from build123d import *

# Parameters (mm, degrees)
EXTRUDE7_START     = 10
SKETCH1_R          = 2.25
SKETCH1_R_2        = 14.05
EXTRUDE7_DEPTH     = 30
CUT_EXTRUDE6_START = 2
SKETCH8_R          = 2.25
CUT_EXTRUDE6_DEPTH = 30


with BuildPart() as part:
    # Sketch1 → Extrude7 (new body)
    with BuildSketch(Plane.XY.offset(EXTRUDE7_START)):
        Polygon((20, 44), (-20, 44), (-22, 44), (-22, -44), (-20, -44), (20, -44), align=None)
        with Locations((-13.435028843, -13.435028843)):
            Circle(SKETCH1_R, mode=Mode.SUBTRACT)
        with Locations((0, -19)):
            Circle(SKETCH1_R, mode=Mode.SUBTRACT)
        with Locations((13.435028843, -13.435028843)):
            Circle(SKETCH1_R, mode=Mode.SUBTRACT)
        with Locations((-13.435028843, 13.435028843)):
            Circle(SKETCH1_R, mode=Mode.SUBTRACT)
        Circle(SKETCH1_R_2, mode=Mode.SUBTRACT)
        with Locations((0, 19)):
            Circle(SKETCH1_R, mode=Mode.SUBTRACT)
        with Locations((13.435028843, 13.435028843)):
            Circle(SKETCH1_R, mode=Mode.SUBTRACT)
        Polygon((20, 44), (-20, 44), (-22, 44), (-22, -44), (-20, -44), (20, -44), align=None)
        with Locations((-13.435028843, -13.435028843)):
            Circle(SKETCH1_R, mode=Mode.SUBTRACT)
        with Locations((0, -19)):
            Circle(SKETCH1_R, mode=Mode.SUBTRACT)
        with Locations((13.435028843, -13.435028843)):
            Circle(SKETCH1_R, mode=Mode.SUBTRACT)
        with Locations((-13.435028843, 13.435028843)):
            Circle(SKETCH1_R, mode=Mode.SUBTRACT)
        Circle(SKETCH1_R_2, mode=Mode.SUBTRACT)
        with Locations((0, 19)):
            Circle(SKETCH1_R, mode=Mode.SUBTRACT)
        with Locations((13.435028843, 13.435028843)):
            Circle(SKETCH1_R, mode=Mode.SUBTRACT)
        Polygon((20, 44), (-20, 44), (-22, 44), (-22, -44), (-20, -44), (20, -44), align=None)
        with Locations((-13.435028843, -13.435028843)):
            Circle(SKETCH1_R, mode=Mode.SUBTRACT)
        with Locations((0, -19)):
            Circle(SKETCH1_R, mode=Mode.SUBTRACT)
        with Locations((13.435028843, -13.435028843)):
            Circle(SKETCH1_R, mode=Mode.SUBTRACT)
        with Locations((-13.435028843, 13.435028843)):
            Circle(SKETCH1_R, mode=Mode.SUBTRACT)
        Circle(SKETCH1_R_2, mode=Mode.SUBTRACT)
        with Locations((0, 19)):
            Circle(SKETCH1_R, mode=Mode.SUBTRACT)
        with Locations((13.435028843, 13.435028843)):
            Circle(SKETCH1_R, mode=Mode.SUBTRACT)
    extrude(amount=EXTRUDE7_DEPTH)

    # Sketch8 → Cut-Extrude6 (cut)
    with BuildSketch(Plane.ZY.offset(20).offset(CUT_EXTRUDE6_START)):
        with Locations((17.5, 39)):
            Circle(SKETCH8_R)
        with Locations((32.5, 39)):
            Circle(SKETCH8_R)
        with Locations((17.5, -39)):
            Circle(SKETCH8_R)
        with Locations((32.5, -39)):
            Circle(SKETCH8_R)
        with Locations((17.5, 29)):
            Circle(SKETCH8_R)
        with Locations((32.5, 29)):
            Circle(SKETCH8_R)
        with Locations((17.5, -29)):
            Circle(SKETCH8_R)
        with Locations((32.5, -29)):
            Circle(SKETCH8_R)
    extrude(amount=-CUT_EXTRUDE6_DEPTH, mode=Mode.SUBTRACT)


solid = part.part
Work out the finished part from the listing and answer in its coordinate system (mm). A direction names the side the tool comes from. Coordinates: 2 decimals unless noted, no trailing zeros. Write each loop counter-clockwise with the first axis right and the second up, starting at its lowest first coordinate (ties: lowest second). Pieces come first, ordered by that corner, then holes. Notation, with made-up numbers: M -7,-4.5 L 8,-4.5 A25 cw 8,34.5 Z; hole C 79,1.5 d6. An arc over 180 degrees is marked long. Write item = value, one per line.
1. Flat-ended cylindrical pins translate along their axes: pin 1 (4 mm diameter, centred on x = 13.44, y = -13.44, fed in from -Z); pin 2 (2.5 mm diameter, centred on y = 29, z = 17.5, fed in from -X). Find the tip coordinate at first contact, or state that the pin passes through.
Solution:
pin_1 = through
pin_2 = 8
2. The part is cut by section A-A (y = 19). Determine the outline of the cut face in (x, z).
Solution:
outline = M -22,10 L -2.25,10 L -2.25,40 L -22,40 Z; M 2.25,10 L 20,10 L 20,40 L 2.25,40 Z
3. For faces 4 (the face through (8, 39, 32)), 5 (the face through (14.473, 11.439, 24.79)), determine the directions among +Z, -Z, +X, -X, +Y, -Y from which every point of the face is accessible in a straight line to the end or side of a thin tool.
Solution:
face_4 = -X
face_5 = +Z, -Z
4. Determine the mould class of faces 1 (the face through (-22, 1, 25)), 2 (the face through (-11.29, -12.76, 24.79)), 3 (the face through (-7.21, 40.897, 33.71)) for opening direction X: released by +X, released by -X, zero draft, split by the parting line, or undercut.
Solution:
face_1 = released by -X
face_2 = undercut
face_3 = zero draft
5. The part is cut by section B-B (x = -4). State how many separate pieces and enclosed holes the cut face has, then the cut area to 3 significant figures.
Solution:
separate_pieces = 2
enclosed_holes = 8
area = 1,700 mm2
6. Straight lines are drawn through the part: line 1 (Y direction, x = 0, z = 28); line 2 (Y direction, x = -6.25, z = 32.5); line 3 (Y direction, x = 4, z = 19.5). For each, find the intervals that lie inside material, in ascending order. Write a range as from..to.
Solution:
line_1 = -44..-21.25, -16.75..-14.05, 14.05..16.75, 21.25..44
line_2 = -44..-41.25, -36.75..-31.25, -26.75..-12.58, 12.58..26.75, 31.25..36.75, 41.25..44
line_3 = -44..-40.03, -37.97..-30.03, -27.97..-13.47, 13.47..27.97, 30.03..37.97, 40.03..44
7. The part is cut by section D-D (y = -39). Determine the outline of the cut face in (x, z), then the cut area to 3 significant figures.
Solution:
outline = M -22,10 L 20,10 L 20,40 L -22,40 L -22,34.75 L 8,34.75 L 8,30.25 L -22,30.25 L -22,19.75 L 8,19.75 L 8,15.25 L -22,15.25 Z
area = 990 mm2
8. The part is cut by section C-C (z = 32.25). Determine the outline of the cut face in (x, y), then the cut area to 3 significant figures.
Solution:
outline = M -22,-44 L 20,-44 L 20,44 L -22,44 L -22,41.24 L 8,41.24 L 8,36.76 L -22,36.76 L -22,31.24 L 8,31.24 L 8,26.76 L -22,26.76 L -22,-26.76 L 8,-26.76 L 8,-31.24 L -22,-31.24 L -22,-36.76 L 8,-36.76 L 8,-41.24 L -22,-41.24 Z; hole C -13.44,-13.44 d4.5; hole C -13.44,13.44 d4.5; hole C 0,0 d28.1; hole C 0,-19 d4.5; hole C 0,19 d4.5; hole C 13.44,-13.44 d4.5; hole C 13.44,13.44 d4.5
area = 2,440 mm2
